from build123d import *

# Parameters (mm, degrees)
BOSS_EXTRUDE1_DEPTH = 11.8
BOSS_EXTRUDE2_DEPTH = 4
SKETCH3_R           = 2.3
CUT_EXTRUDE1_DEPTH  = 4
CUT_EXTRUDE2_DEPTH  = 4


with BuildPart() as part:
    # Sketch1 → Boss-Extrude1 (new body)
    with BuildSketch(Plane.XY):
        Polygon((0, 0), (22.5, 0), (22.5, 15.9), (27.2, 15.9), (27.2, 18.4), (22.5, 18.4), (22.5, 22.7), (0, 22.7), (0, 18.4), (-4.7, 18.4), (-4.7, 15.9), (0, 15.9), align=None)
    extrude(amount=BOSS_EXTRUDE1_DEPTH)

    # Sketch2 → Boss-Extrude2 (add)
    with BuildSketch(Plane(origin=(0, 22.7, 0), x_dir=(1, 0, 0), z_dir=(0, 1, 0))):
        with BuildLine():
            Line((12.2, -3.4), (11.244155686, -3.4))
            ThreePointArc((11.244155686, -3.4), (0, -5.9), (11.244155686, -8.4))
            Line((11.244155686, -8.4), (12.2, -8.4))
            ThreePointArc((12.2, -8.4), (14.7, -5.9), (12.2, -3.4))
        make_face()
    extrude(amount=BOSS_EXTRUDE2_DEPTH)

    # Sketch3 → Cut-Extrude1 (cut)
    with BuildSketch(Plane(origin=(0, 26.7, 0), x_dir=(1, 0, 0), z_dir=(0, 1, 0))):
        with Locations(Location((5.9, -5.9, 0), (0, 0, 270))):
            Circle(SKETCH3_R)
    extrude(amount=-CUT_EXTRUDE1_DEPTH, mode=Mode.SUBTRACT)

    # Sketch4 → Cut-Extrude2 (cut)
    with BuildSketch(Plane(origin=(0, 18.4, 0), x_dir=(1, 0, 0), z_dir=(0, 1, 0))):
        with BuildLine():
            Line((-4.7, -5.25), (-4.7, -6.55))
            Line((-4.7, -6.55), (-3.109934208, -6.55))
            ThreePointArc((-3.109934208, -6.55), (-1.35, -5.9), (-3.109934208, -5.25))
            Line((-3.109934208, -5.25), (-4.7, -5.25))
        make_face()
    cut_extrude2 = extrude(amount=-CUT_EXTRUDE2_DEPTH, mode=Mode.SUBTRACT)

    # Mirror1: Cut-Extrude2 across plane
    add(cut_extrude2.mirror(Plane(origin=(11.25, 0, 0), x_dir=(0, 0, 1), z_dir=(1, 0, 0))), mode=Mode.SUBTRACT)


solid = part.part
Work out the finished part from the listing and answer in its coordinate system (mm). A direction names the side the tool comes from. Give positions to 0.01 mm unless a question says otherwise; leave off trailing zeros. Order: outer loops, then holes, each group sorted by start corner. A loop starts at its lowest first (then second) coordinate and runs counter-clockwise, first axis right, second up. Notation, with made-up numbers: (60.25, -21) -> (74.25, -21) arc R19 ccw to (74.25, 3) -> close; hole circle Ø5 at (-24, 4). An arc over 180 degrees is marked (long way). Answer as a JSON object with one key per item and string values. Group by question number.
1. Section B-B on z = 4.5 is taken. Determine the outline of the cut face in (x, y), plus the area to 3 significant figures.
2. A tool of negligible diameter and unlimited length cuts with its end or side. For faces 1 (the flat face through (0, 21, 6)), 2 (the flat face through (16, 22.7, 6)), 3 (the flat face through (12, 25, 8.4)), 4 (the flat face through (0, 8, 6)), from which of +Z, -Z, +X, -X, +Y, -Y can it reach the whole face along a straight path? Write none if from no direction.
3. The mould has two halves that part along Z. Classify faces 5 (the flat face through (27.2, 17, 3)), 6 (the flat face through (11, 12, 11.8)), 7 (the flat face through (-4, 17, 6.55)): released by +Z, released by -Z, zero draft, split by the parting line, or undercut.
4. Section D-D on x = 21 is taken. Determine the outline of the cut face in (y, z), plus the area to 3 significant figures.
5. Consider line 1 along X through (y, z) = (25.45, 5.9); line 2 along Z through (x, y) = (24.85, 17.5); line 3 along Y through (x, z) = (24, 9.5). Determine where each line is inside the solid, lowest interval first. Write a range as [from, to].
6. Section C-C on y = 21 is taken. Determine the outline of the cut face in (x, z).
7. Flat-ended cylindrical pins translate along their axes: pin 1 Ø0.8 at (x, y) = (11.5, 24) entering from +Z; pin 2 Ø1 at (y, z) = (23, 2) entering from +X; pin 3 Ø2.5 at (x, z) = (-3, 6) entering from -Y. Find the tip coordinate at first contact, or state that the pin passes through.
8. Section A-A on x = -2.35 is taken. Determine the outline of the cut face in (y, z).
Result sheet:
{
 "1": {"outline": "(-4.7, 15.9) -> (0, 15.9) -> (0, 0) -> (22.5, 0) -> (22.5, 15.9) -> (27.2, 15.9) -> (27.2, 18.4) -> (22.5, 18.4) -> (22.5, 22.7) -> (14.27, 22.7) -> (14.27, 26.7) -> (7.72, 26.7) -> (7.72, 22.7) -> (4.08, 22.7) -> (4.08, 26.7) -> (0.17, 26.7) -> (0.17, 22.7) -> (0, 22.7) -> (0, 18.4) -> (-4.7, 18.4) -> close", "area": "576 mm^2"},
 "2": {"face 1": "+Z, -Z, -X, +Y", "face 2": "+X, +Y", "face 3": "+Z, +X, +Y", "face 4": "+Z, -Z, -X, -Y"},
 "3": {"face 5": "zero draft", "face 6": "released by +Z", "face 7": "undercut"},
 "4": {"outline": "(0, 0) -> (22.7, 0) -> (22.7, 11.8) -> (0, 11.8) -> close", "area": "268 mm^2"},
 "5": {"line 1": "x = [0, 3.6], [8.2, 14.7]", "line 2": "z = [0, 4.9], [6.9, 11.8]", "line 3": "y = [15.9, 18.4]"},
 "6": {"outline": "(0, 0) -> (22.5, 0) -> (22.5, 11.8) -> (0, 11.8) -> close"},
 "7": {"pin 1": "stops at z = 8.69", "pin 2": "stops at x = 22.5", "pin 3": "stops at y = 15.9"},
 "8": {"outline": "(15.9, 0) -> (18.4, 0) -> (18.4, 4.9) -> (15.9, 4.9) -> close; (15.9, 6.9) -> (18.4, 6.9) -> (18.4, 11.8) -> (15.9, 11.8) -> close"}
}
